Part model, mm, in its own coordinate system. A direction names the side the tool comes from. Round coordinates to 2 decimals unless told otherwise and drop trailing zeros. Loops run counter-clockwise (first coordinate to the right, second up) from the corner with the lowest first, then second, coordinate; pieces in that order, holes last. Notation, with made-up numbers: (59, -2.75) -> (89, -2.75) arc R11 cw to (89, 3.25) -> close; hole circle Ø6 at (79, 76). An arc over 180 degrees is marked (long way). Answer as a JSON object with one key per item and string values. Group by question number.
from build123d import *

# Parameters (mm, degrees)
BOSS_EXTRU_1_DEPTH      = 10
ESQUISSE2_R             = 2.5
ENL_V_MAT_EXTRU_1_DEPTH = 8


with BuildPart() as part:
    # Esquisse1 → Boss.-Extru.1 (new, symmetric)
    with BuildSketch(Plane.XY):
        with BuildLine():
            Line((46.618888989, 57.076719782), (101.618888989, 57.076719782))
            Line((101.618888989, 57.076719782), (48.527534404, 79.003668292))
            ThreePointArc((48.527534404, 79.003668292), (43.838891424, 78.538210075), (41.618888989, 74.382296994))
            Line((41.618888989, 74.382296994), (41.618888989, 62.076719782))
            ThreePointArc((41.618888989, 62.076719782), (43.083355083, 58.541185876), (46.618888989, 57.076719782))
        make_face()
        with BuildLine():
            Line((72.136693702, 64.925268301), (50.45494078, 73.879921722))
            ThreePointArc((50.45494078, 73.879921722), (47.172890694, 73.554100969), (45.618888989, 70.644961813))
            Line((45.618888989, 70.644961813), (45.618888989, 64.576719782))
            ThreePointArc((45.618888989, 64.576719782), (46.644015255, 62.101846047), (49.118888989, 61.076719782))
            Line((49.118888989, 61.076719782), (71.373235536, 61.076719782))
            Line((71.373235536, 61.076719782), (82.169018373, 61.076719782))
            Line((82.169018373, 61.076719782), (72.136693702, 64.925268301))
        make_face(mode=Mode.SUBTRACT)
    extrude(amount=BOSS_EXTRU_1_DEPTH, both=True)

    # Esquisse2 → Enlèv. mat.-Extru.1 (cut)
    with BuildSketch(Plane(origin=(34.945552376, 84.613082912, 0), x_dir=(0.9242742597143897, -0.38172908302802533, 0), z_dir=(0.3817290830280253, 0.9242742597143896, 0))):
        with Locations(Location((21.875034686, 0, 0), (0, 0, 180))):
            Circle(ESQUISSE2_R)
        with Locations(Location((36.235316287, 0, 0), (0, 0, 180))):
            Circle(ESQUISSE2_R)
    extrude(amount=-ENL_V_MAT_EXTRU_1_DEPTH, mode=Mode.SUBTRACT)


solid = part.part
Item 1: Drop flat-ended pins along their axis: pin 1 Ø12 at (x, y) = (81, 67) entering from +Z; pin 2 Ø6.5 at (y, z) = (68, -1) entering from +X; pin 3 Ø1 at (x, z) = (62, 5.5) entering from +Y; pin 4 Ø10 at (x, z) = (57.5, 6) entering from +Y. Give the stop position or say it passes through.
Item 2: Two-plate mould, pull along X, no slides. Class faces 3 (the face through (43.9, 78.58, 0.14)), 4 (the face through (45.619, 68, 0)), 5 (the face through (43.045, 58.58, 0.14)), 6 (the face through (61.45, 69.34, 0.14)): pulls with the +X half, pulls with the -X half, needs draft (parallel to the pull), parting line crosses it, or undercut.
Item 3: Drill centre lines: line 1 (X direction, y = 68.5, z = 0.5); line 2 (Y direction, x = 66, z = -2.5); line 3 (Y direction, x = 52.5, z = 0.75). Where is each one in solid material? Low to high.
Item 4: Band-saw the part on C-C, the plane y = 69.5. Count the separate pieces of the cut face and the enclosed holes in it, plus the area to 3 significant figures.
Item 5: Which spindle directions (+Z, -Z, +X, -X, +Y, -Y) get a long thin tool onto all of the face, cutting with end or side? Do faces 1 (the face through (69.99, 68, 0.11)), 2 (the face through (65, 61.077, 0)). Say none if no direction does.
Item 6: Band-saw the part on A-A, the plane z = 7.25. List the corners of the cut face in (x, y).
Item 7: Band-saw the part on D-D, the plane x = 89.5. List the corners of the cut face in (y, z), plus the area to 3 significant figures.
Item 8: Band-saw the part on B-B, the plane x = 81.5. List the corners of the cut face in (y, z).
Entries:
{
 "1": {"pin 1": "z = 10", "pin 2": "x = 83.04", "pin 3": "y = 73.65", "pin 4": "y = 77.36"},
 "2": {"face 3": "parting line crosses it", "face 4": "undercut", "face 5": "pulls with the -X half", "face 6": "undercut"},
 "3": {"line 1": "41.62 to 45.62, 63.48 to 64.84, 70.15 to 73.96", "line 2": "57.08 to 61.08, 67.46 to 71.79", "line 3": "57.08 to 61.08, 76.06 to 77.36"},
 "4": {"separate pieces": "2", "enclosed holes": "1", "area": "268 mm²"},
 "5": {"face 1": "none", "face 2": "+Z, -Z"},
 "6": {"outline": "(41.62, 62.08) arc R5 ccw to (46.62, 57.08) -> (101.62, 57.08) -> (48.53, 79) arc R5 ccw to (41.62, 74.38) -> close; hole (45.62, 64.58) arc R3.5 ccw to (49.12, 61.08) -> (82.17, 61.08) -> (72.14, 64.93) -> (50.45, 73.88) arc R3.5 ccw to (45.62, 70.64) -> close"},
 "7": {"outline": "(57.08, -10) -> (62.08, -10) -> (62.08, 10) -> (57.08, 10) -> close", "area": "100 mm²"},
 "8": {"outline": "(57.08, -10) -> (61.08, -10) -> (61.08, 10) -> (57.08, 10) -> close; (61.33, -10) -> (65.39, -10) -> (65.39, 10) -> (61.33, 10) -> close"}
}
